```python
from build123d import *

# Parameters (mm, degrees)
SKETCH_1_W      = 15
SKETCH_1_H      = 10.5
EXTRUDE_1_DEPTH = 1.4
EXTRUDE_2_DEPTH = 6.194784772
SKETCH_3_W      = 13.5
SKETCH_3_H      = 9
EXTRUDE_3_DEPTH = 9.6
SKETCH_4_W      = 1.830527318
SKETCH_4_H      = 5
EXTRUDE_4_DEPTH = 0.3
SKETCH_5_W      = 0.5
SKETCH_5_H      = 3.7
EXTRUDE_5_DEPTH = 5
SKETCH_6_W      = 1.830527318
SKETCH_6_H      = 5
EXTRUDE_6_DEPTH = 0.3
SKETCH_7_W      = 0.5
SKETCH_7_H      = 3.7
EXTRUDE_7_DEPTH = 5
DRAFT_1_ANGLE   = 26
FILLET_1_R      = 0.6


with BuildPart() as part:
    # 草图1 → 凸台-拉伸1 (new body)
    with BuildSketch(Plane.XY.offset(11)):
        Rectangle(SKETCH_1_W, SKETCH_1_H)
    extrude(amount=-EXTRUDE_1_DEPTH)

    # 草图2 → 凸台-拉伸2 (add)
    with BuildSketch(Plane.XZ.offset(3.097392386)):
        Polygon((5.416790428, 11), (5.416790428, 13.171623136), (-5.441325251, 11), align=None)
    extrude(amount=-EXTRUDE_2_DEPTH)

    # 草图3 → 凸台-拉伸3 (add)
    with BuildSketch(Plane(origin=(0, 0, 9.6), x_dir=(-1, 0, 0), z_dir=(0, 0, -1))):
        Rectangle(SKETCH_3_W, SKETCH_3_H)
    extrude(amount=EXTRUDE_3_DEPTH)

    # 草图4 → 凸台-拉伸4 (add)
    with BuildSketch(Plane(origin=(0, 0, 0), x_dir=(-1, 0, 0), z_dir=(0, 0, -1))):
        Rectangle(SKETCH_4_W, SKETCH_4_H)
    extrude(amount=EXTRUDE_4_DEPTH)

    # 草图5 → 凸台-拉伸5 (add)
    with BuildSketch(Plane(origin=(0, 0, -0.3), x_dir=(-1, 0, 0), z_dir=(0, 0, -1))):
        Rectangle(SKETCH_5_W, SKETCH_5_H)
    extrude(amount=EXTRUDE_5_DEPTH)

    # 草图6 → 凸台-拉伸6 (add)
    with BuildSketch(Plane(origin=(0, 0, 0), x_dir=(-1, 0, 0), z_dir=(0, 0, -1))):
        with Locations((-4.709769509, 0)):
            Rectangle(SKETCH_6_W, SKETCH_6_H)
    extrude(amount=EXTRUDE_6_DEPTH)

    # 草图7 → 凸台-拉伸7 (add)
    with BuildSketch(Plane(origin=(0, 0, -0.3), x_dir=(-1, 0, 0), z_dir=(0, 0, -1))):
        with Locations((-4.709769509, 0)):
            Rectangle(SKETCH_7_W, SKETCH_7_H)
    extrude(amount=EXTRUDE_7_DEPTH)

    # 拔模1
    draft_1_faces = [part.faces().sort_by_distance(p)[0] for p in [
        (5.416790428, 0, 12.085811568),
    ]]
    draft(draft_1_faces, Plane.XY.offset(11), DRAFT_1_ANGLE)

    # 圆角1
    fillet_1_edges = [part.edges().sort_by_distance(p)[0] for p in [
        (7.5, 0, 11),
        (0, -5.25, 11),
        (-7.5, 0, 11),
        (0, 5.25, 11),
    ]]
    fillet(fillet_1_edges, radius=FILLET_1_R)


solid = part.part
```
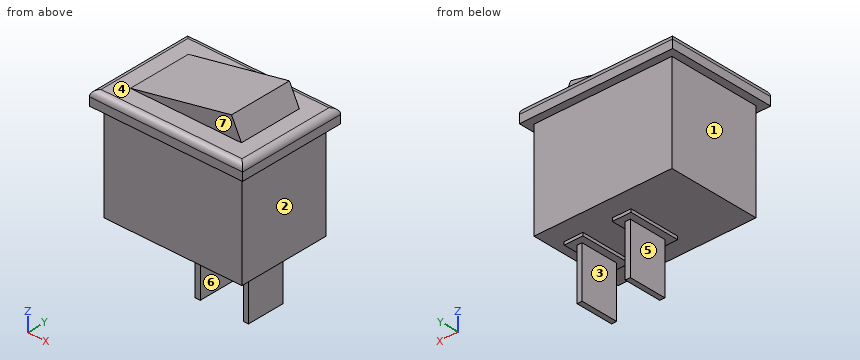
Could you check a few things on this model? Use its own coordinates, in mm. Face numbers are marked on the shaded views. A direction names the side the tool comes from. Round coordinates to 2 decimals unless told otherwise and drop trailing zeros. Loops run counter-clockwise (first coordinate to the right, second up) from the corner with the lowest first, then second, coordinate; pieces in that order, holes last. Notation, with made-up numbers: (67.5, 42.25) - (80.5, 42.25) arc R29 ccw to (80.5, 67.25) - close; hole circle Ø3 at (52, 12). An arc over 180 degrees is marked (long way). Use CSV: the item, a comma, the result in double quotes.
Item 1: If we section it at D-D on z = 1.5: List the corners of the cut face in (x, y) for me.
Here are the results:
outline,"(-6.75, -4.5) - (6.75, -4.5) - (6.75, 4.5) - (-6.75, 4.5) - close"
Item 2: If we section it at B-B on y = -2.25: List the corners of the cut face in (x, z) for me.
Here are the results:
outline,"(-7.5, 9.6) - (-6.75, 9.6) - (-6.75, 0) - (-0.92, 0) - (-0.92, -0.3) - (0.92, -0.3) - (0.92, 0) - (3.79, 0) - (3.79, -0.3) - (5.63, -0.3) - (5.63, 0) - (6.75, 0) - (6.75, 9.6) - (7.5, 9.6) - (7.5, 10.4) arc R0.6 ccw to (6.9, 11) - (5.42, 11) - (4.45, 12.98) - (-5.44, 11) - (-6.9, 11) arc R0.6 ccw to (-7.5, 10.4) - close"
Item 3: I need wall thicknesses on L1, parallel to X at y = 0.5, z = -1.5; L2, parallel to X at y = 3, z = 0.5; L3, parallel to Y at x = 1.25, z = 3.75. Which ranges of each line are inside material? Lowest first, please. Write a range as [from, to].
Here are the results:
L1,"x = [-0.25, 0.25], [4.46, 4.96]"
L2,"x = [-6.75, 6.75]"
L3,"y = [-4.5, 4.5]"
Item 4: If we section it at C-C on x = -6.25: List the corners of the cut face in (y, z) for me.
Here are the results:
outline,"(-5.25, 9.6) - (-4.5, 9.6) - (-4.5, 0) - (4.5, 0) - (4.5, 9.6) - (5.25, 9.6) - (5.25, 10.4) arc R0.6 ccw to (4.65, 11) - (-4.65, 11) arc R0.6 ccw to (-5.25, 10.4) - close"
Item 5: If we section it at A-A on z = -2.25: List the corners of the cut face in (x, y) for me, then the cut area to 3 significant figures.
Here are the results:
outline,"(-0.25, -1.85) - (0.25, -1.85) - (0.25, 1.85) - (-0.25, 1.85) - close; (4.46, -1.85) - (4.96, -1.85) - (4.96, 1.85) - (4.46, 1.85) - close"
area,"3.70 mm²"
Item 6: Will these pins go through, and if not, where does the flat tip stop? pin 1 (1.6 mm diameter, centred on x = 2, z = 12, fed in from -Y); pin 2 (6 mm diameter, centred on x = -4.5, y = -4, fed in from -Z); pin 3 (4 mm diameter, centred on y = 0.5, z = -0.5, fed in from -X).
Here are the results:
pin 1,"stops at y = -3.1"
pin 2,"stops at z = 0"
pin 3,"stops at x = -6.75"
Item 7: For the marked faces 4, 5, 6 and 7, which set-ups out of +Z, -Z, +X, -X, +Y, -Y let a thin tool reach every point of the face, with its end or its side?
Here are the results:
face 4,"+Z"
face 5,"-Z, -X, +Y, -Y"
face 6,"-Z, +Y, -Y"
face 7,"+Z, +X, -X, -Y"
Item 8: If we mould it in two halves opening along X, with no side actions, what happens to the marked faces 1, 2 and 3? For each: pulls with the +X half, pulls with the -X half, needs draft (parallel to the pull), parting line crosses it, or undercut.
Here are the results:
face 1,"pulls with the -X half"
face 2,"pulls with the +X half"
face 3,"undercut"
